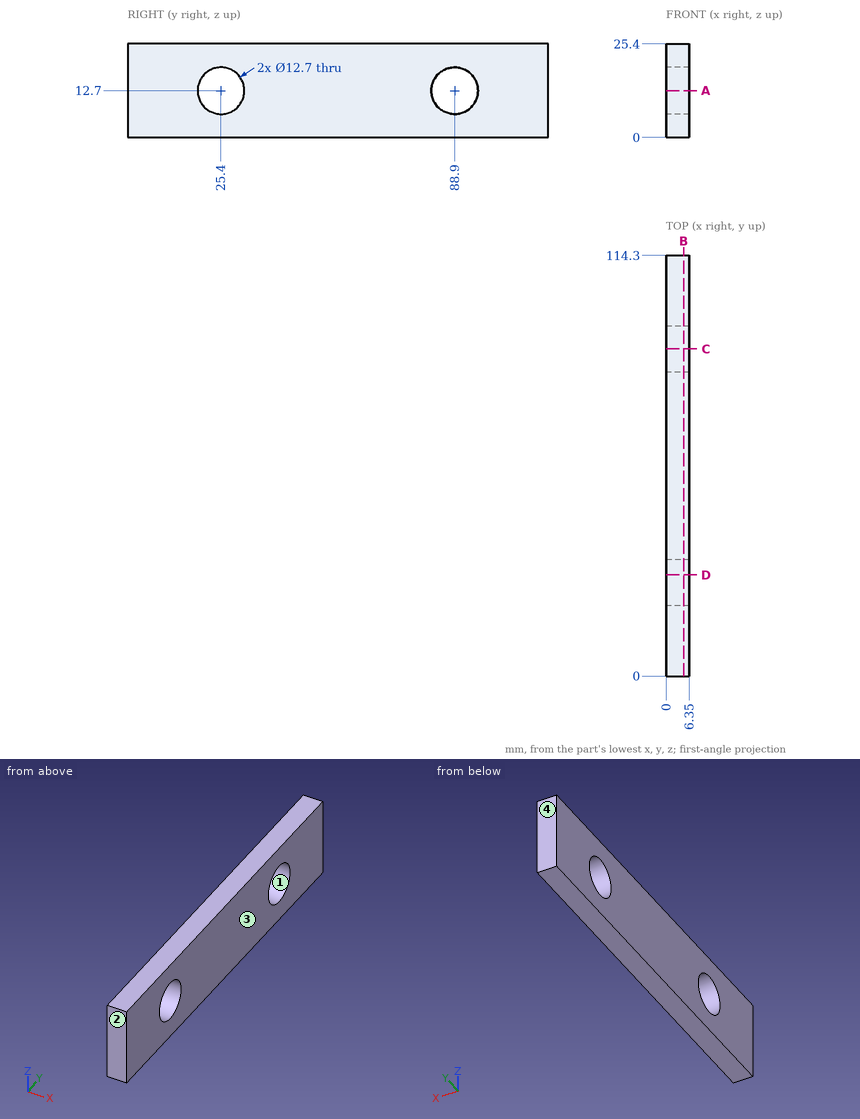
Here's the drawing with two shaded views (mm, measured from the low corner). I have some questions. Round coordinates to 2 decimals unless told otherwise and drop trailing zeros. Order: outer loops, then holes, each group sorted by start corner. A loop starts at its lowest first (then second) coordinate and runs counter-clockwise, first axis right, second up. Notation, with made-up numbers: (51.5, -30) -> (69.5, -30) arc R19 ccw to (69.5, -10) -> close; hole circle Ø2 at (89, -11.75). An arc over 180 degrees is marked (long way). Use a Markdown table: item, result. Add a question column.
(1) I need wall thicknesses on line 1 along Z through (x, y) = (3, 25.4); line 2 along Y through (x, z) = (3, 9.25); line 3 along Y through (x, z) = (6.25, 11.25). Which ranges of each line are inside material? Lowest first, please.
(2) Suppose I cut it at C-C, the plane y = 88.9. Please give me the cut outline in (x, z), and give its area (3 significant figures).
(3) If we mould it in two halves opening along Y, with no side actions, what happens to the marked faces 1, 2, 3 and 4? For each: released by +Y, released by -Y, zero draft, split by the parting line, or undercut.
(4) Suppose I cut it at B-B, the plane x = 4.75. Please give me the cut outline in (y, z), and give its area (3 significant figures).
(5) Suppose I cut it at D-D, the plane y = 27.5. Please give me the cut outline in (x, z), and give its area (3 significant figures).
(6) For pin 1 Ø11.5 at (y, z) = (25.4, 12.7) entering from -X, with a flat end and sliding along its axis, tell me the tip position at first contact or that it passes through.
(7) Suppose I cut it at A-A, the plane z = 12.7. Please give me the cut outline in (x, y), and give its area (3 significant figures).
Verdict:
| question | item | result |
|---|---|---|
| 1 | line 1 | 0 to 6.35, 19.05 to 25.4 |
| 1 | line 2 | 0 to 20.07, 30.73 to 83.57, 94.23 to 114.3 |
| 1 | line 3 | 0 to 19.22, 31.58 to 82.72, 95.08 to 114.3 |
| 2 | outline | (0, 0) -> (6.35, 0) -> (6.35, 6.35) -> (0, 6.35) -> close; (0, 19.05) -> (6.35, 19.05) -> (6.35, 25.4) -> (0, 25.4) -> close |
| 2 | area | 80.6 mm2 |
| 3 | face 1 | undercut |
| 3 | face 2 | released by -Y |
| 3 | face 3 | zero draft |
| 3 | face 4 | released by +Y |
| 4 | outline | (0, 0) -> (114.3, 0) -> (114.3, 25.4) -> (0, 25.4) -> close; hole circle Ø12.7 at (25.4, 12.7); hole circle Ø12.7 at (88.9, 12.7) |
| 4 | area | 2,650 mm2 |
| 5 | outline | (0, 0) -> (6.35, 0) -> (6.35, 6.71) -> (0, 6.71) -> close; (0, 18.69) -> (6.35, 18.69) -> (6.35, 25.4) -> (0, 25.4) -> close |
| 5 | area | 85.2 mm2 |
| 6 | pin 1 | through |
| 7 | outline | (0, 0) -> (6.35, 0) -> (6.35, 19.05) -> (0, 19.05) -> close; (0, 31.75) -> (6.35, 31.75) -> (6.35, 82.55) -> (0, 82.55) -> close; (0, 95.25) -> (6.35, 95.25) -> (6.35, 114.3) -> (0, 114.3) -> close |
| 7 | area | 565 mm2 |
